Input: dimensioned drawing with shaded views. Units: mm. Origin: part minimum x, y, z. A direction names the side the tool comes from. Give positions to 0.01 mm unless a question says otherwise; leave off trailing zeros. Loops run counter-clockwise (first coordinate to the right, second up) from the corner with the lowest first, then second, coordinate; pieces in that order, holes last.
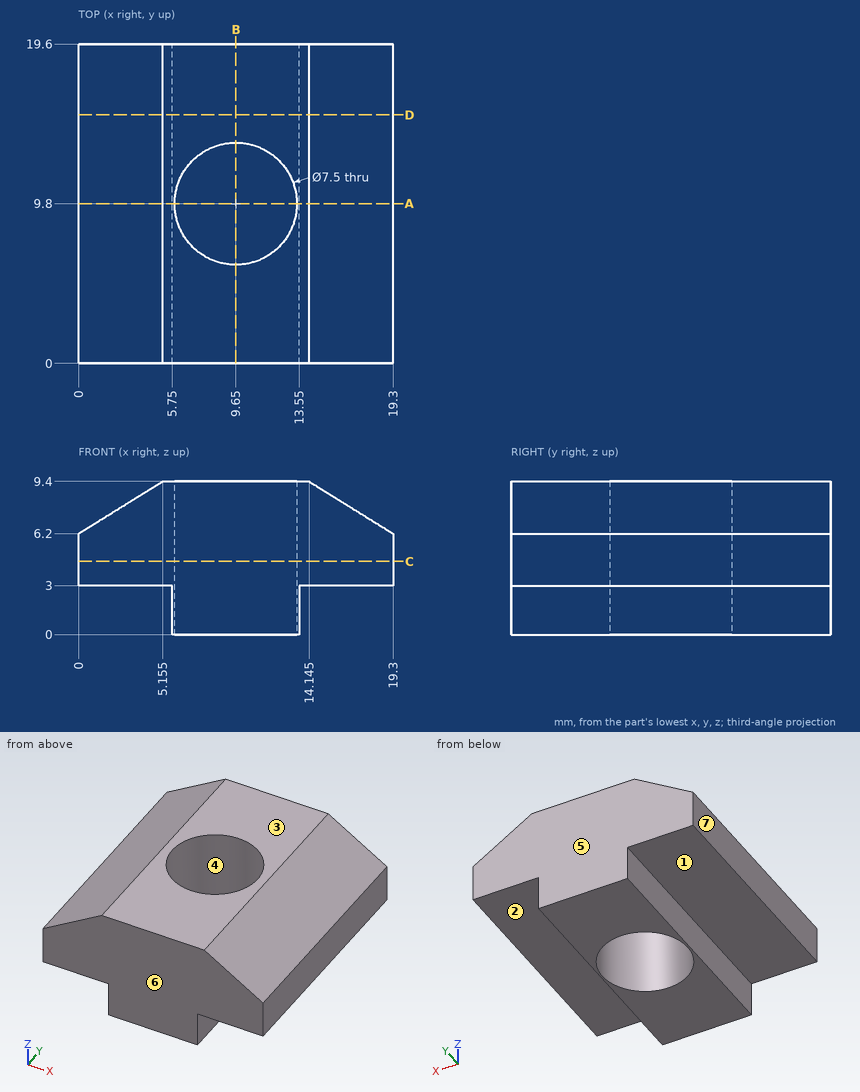
Item 1: Set-up query: the marked faces 1, 2 and 3. Return all of +Z, -Z, +X, -X, +Y, -Y with unobstructed straight access to the full face (end or side cutting, diameter ignored); none if empty.
Values follow:
face 1: -Z, -X, +Y, -Y
face 2: -Z, +X, +Y, -Y
face 3: +Z, +X, -X, +Y, -Y
Item 2: Section query C-C on z = 4.5. Return loops of the section in (x, y).
Values follow:
outline: (0, 0) - (19.3, 0) - (19.3, 19.6) - (0, 19.6) - close; hole circle Ø7.5 at (9.65, 9.8)
Item 3: Pin query (flat end, axial travel): pin 1 (1.5 mm diameter, centred on y = 5, z = 1, fed in from +X); pin 2 (6 mm diameter, centred on x = 9.65, y = 9.8, fed in from +Z); pin 3 (1.5 mm diameter, centred on y = 6.5, z = 1.5, fed in from -X); pin 4 (6.5 mm diameter, centred on x = 17.5, y = 9, fed in from -Z). Return the tip coordinate at first contact, or that it passes through.
Values follow:
pin 1: stops at x = 13.55
pin 2: passes through
pin 3: stops at x = 5.75
pin 4: stops at z = 3
Item 4: Section query D-D on y = 15.25. Return loops of the section in (x, z) (3 decimals).
Values follow:
outline: (0, 3) - (5.75, 3) - (5.75, 0) - (13.55, 0) - (13.55, 3) - (19.3, 3) - (19.3, 6.2) - (14.145, 9.4) - (5.155, 9.4) - (0, 6.2) - close
Item 5: Draft query along Y for the marked faces 4, 5, 6 and 7. Return one class per face: +Y half, -Y half, draft (parallel to the pull), parting line (faces both ways), or undercut.
Values follow:
face 4: undercut
face 5: +Y half
face 6: -Y half
face 7: draft
Item 6: Section query A-A on y = 9.8. Return loops of the section in (x, z) (3 decimals).
Values follow:
outline: (0, 3) - (5.75, 3) - (5.75, 0) - (5.9, 0) - (5.9, 9.4) - (5.155, 9.4) - (0, 6.2) - close; (13.4, 0) - (13.55, 0) - (13.55, 3) - (19.3, 3) - (19.3, 6.2) - (14.145, 9.4) - (13.4, 9.4) - close
Item 7: Section query B-B on x = 9.65. Return loops of the section in (y, z).
Values follow:
outline: (0, 0) - (6.05, 0) - (6.05, 9.4) - (0, 9.4) - close; (13.55, 0) - (19.6, 0) - (19.6, 9.4) - (13.55, 9.4) - close
Item 8: Ray query, probe 1 along Y at (x, z) = (9.65, 4); probe 2 along Z at (x, y) = (13.75, 6.25); probe 3 along Y at (x, z) = (11.75, 6.75). Return the intervals inside material, ascending.
Values follow:
probe 1: y = 0 to 6.05, 13.55 to 19.6
probe 2: z = 3 to 9.4
probe 3: y = 0 to 6.69, 12.91 to 19.6
